Geometry check sheet. Reference: the model listing, model coordinates, mm. Face numbers are marked on the shaded views. A direction names the side the tool comes from. Round coordinates to 2 decimals unless told otherwise and drop trailing zeros. Loops run counter-clockwise (first coordinate to the right, second up) from the corner with the lowest first, then second, coordinate; pieces in that order, holes last. Notation, with made-up numbers: (6.25, -31) -> (24.25, -31) arc R27 cw to (24.25, -3) -> close; hole circle Ø2 at (50.5, 24.5). An arc over 180 degrees is marked (long way). Use a Markdown table: item, result. Add a question column.
Q1. Sectioned sample at A-A, the plane y = 150.75. Enter the section's corners in (x, z), then the cut area to 3 significant figures.
Q2. Sectioned sample at C-C, the plane x = 502.5. Enter the section's corners in (y, z).
Q3. Material ranges on L1, parallel to Z at x = 481.5, y = 149.5; L2, parallel to Y at x = 506, z = -18; L3, parallel to Z at x = 495, y = 142.5, recorded low to high.
Q4. Sectioned sample at B-B, the plane z = 21.5. Enter the section's corners in (x, y).
Q5. Gauge pin test, flat ends, axial feed: P1, Ø8.5, axis at x = 484.35, y = 151, coming from the -Z side; P2, Ø4, axis at x = 524, y = 136.5, coming from the +Z side; P3, Ø2, axis at y = 137, z = -47.5, coming from the +X side; P4, Ø4, axis at x = 522.92, z = -75.05, coming from the +Y side. Record the tip position at first contact, or that the pin passes through.
Q6. Set-up check for the marked faces 1 and 2: record each of +Z, -Z, +X, -X, +Y, -Y from which the full face is reachable in a straight line by a thin tool's end or side.
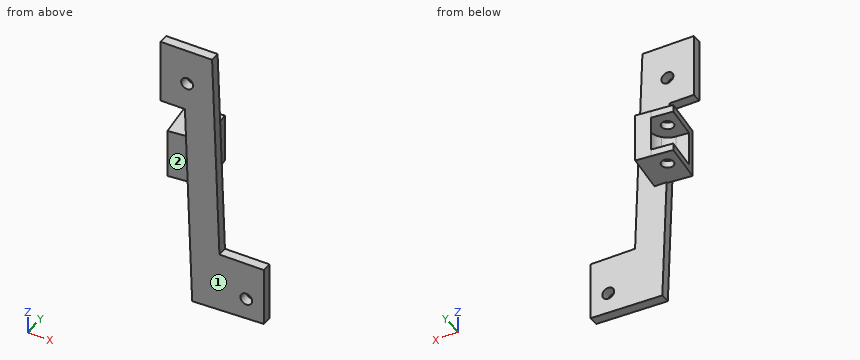
```python
from build123d import *

# Parameters (mm, degrees)
BOSS_EXTRUDE5_DEPTH = 22.352
BOSS_EXTRUDE7_START = -3.81
SKETCH2_R           = 3.175
BOSS_EXTRUDE7_DEPTH = 3.81
BOSS_EXTRUDE8_START = 3.81
SKETCH3_R           = 3.175
BOSS_EXTRUDE8_DEPTH = 3.81
BOSS_EXTRUDE9_DEPTH = 5.08
SKETCH6_R           = 3.175
CUT_EXTRUDE1_DEPTH  = 6.35


with BuildPart() as part:
    # Sketch1 → Boss-Extrude5 (new body)
    with BuildSketch(Plane.XY):
        with BuildLine():
            Line((485.284620904, 141.520479852), (478.661596161, 140.870936716))
            Line((478.661596161, 140.870936716), (479.033472001, 137.079128657))
            Line((479.033472001, 137.079128657), (498.224726786, 138.961281946))
            Line((498.224726786, 138.961281946), (496.114951182, 160.473473003))
            Line((496.114951182, 160.473473003), (488.231748542, 159.700339826))
            ThreePointArc((488.231748542, 159.700339826), (489.092376455, 159.263306748), (489.904354663, 158.741416237))
            ThreePointArc((489.904354663, 158.741416237), (493.83445145, 151.929689602), (491.302607825, 144.484217934))
            ThreePointArc((491.302607825, 144.484217934), (488.563156596, 142.455032775), (485.284620904, 141.520479852))
        make_face()
    extrude(amount=-BOSS_EXTRUDE5_DEPTH)

    # Sketch2 → Boss-Extrude7 (add)
    with BuildSketch(Plane(origin=(0, 0, -22.352), x_dir=(-1, 0, 0), z_dir=(0, 0, -1)).offset(BOSS_EXTRUDE7_START)):
        with BuildLine():
            Line((-476.923696397, 158.591319714), (-478.661596161, 140.870936716))
            Line((-478.661596161, 140.870936716), (-485.284620904, 141.520479852))
            ThreePointArc((-485.284620904, 141.520479852), (-493.757189232, 149.475804861), (-488.231748542, 159.700339826))
            Line((-488.231748542, 159.700339826), (-476.923696397, 158.591319714))
        make_face()
        with Locations(Location((-484.354931302, 151, 0), (0, 0, 90))):
            Circle(SKETCH2_R, mode=Mode.SUBTRACT)
    extrude(amount=BOSS_EXTRUDE7_DEPTH)

    # Sketch3 → Boss-Extrude8 (add)
    # profile 1 of 2: a face of its own
    with BuildSketch(Plane.XY.offset(BOSS_EXTRUDE8_START)):
        with BuildLine():
            Line((488.231748542, 159.700339826), (476.923696397, 158.591319714))
            Line((476.923696397, 158.591319714), (478.661596161, 140.870936716))
            Line((478.661596161, 140.870936716), (485.284620904, 141.520479852))
            ThreePointArc((485.284620904, 141.520479852), (493.757189232, 149.475804861), (488.231748542, 159.700339826))
        make_face()
        with Locations(Location((484.354931302, 151, 0), (0, 0, 90))):
            Circle(SKETCH3_R, mode=Mode.SUBTRACT)
    # profile 2 of 2: a face of its own
    with BuildSketch(Plane.XY.offset(BOSS_EXTRUDE8_START)):
        with BuildLine():
            Line((496.114951182, 160.473473003), (488.231748542, 159.700339826))
            ThreePointArc((488.231748542, 159.700339826), (493.757189232, 149.475804861), (485.284620904, 141.520479852))
            Line((485.284620904, 141.520479852), (478.661596161, 140.870936716))
            Line((478.661596161, 140.870936716), (479.033472001, 137.079128657))
            Line((479.033472001, 137.079128657), (498.224726786, 138.961281946))
            Line((498.224726786, 138.961281946), (496.114951182, 160.473473003))
        make_face()
    extrude(amount=-BOSS_EXTRUDE8_DEPTH)

    # Sketch4 → Boss-Extrude9 (add)
    with BuildSketch(Plane(origin=(0, 138.961281946, 0), x_dir=(1, 0, 0), z_dir=(0, 1, 0))):
        Polygon((494.072487043, 87.311338989), (532.291432121, 85.970092731), (532.291432121, 54.640280545), (508.611718184, 54.640280545), (504.692489504, -57.038529169), (477.269374414, -57.038529169), (477.269374414, -22.86), (490.206161169, -22.86), align=None)
    extrude(amount=-BOSS_EXTRUDE9_DEPTH)

    # Sketch6 → Cut-Extrude1 (cut)
    with BuildSketch(Plane(origin=(0, 138.961281946, 0), x_dir=(1, 0, 0), z_dir=(0, 1, 0))):
        with Locations(Location((491.366130704, -38.105065935, 0), (0, 0, 270))):
            Circle(SKETCH6_R)
        with Locations(Location((522.91714349, 75.049167666, 0), (0, 0, 270))):
            Circle(SKETCH6_R)
    extrude(amount=-CUT_EXTRUDE1_DEPTH, mode=Mode.SUBTRACT)


solid = part.part
```
Values:
| question | item | result |
|---|---|---|
| 1 | outline | (477.69, -22.35) -> (481.19, -22.35) -> (481.19, -18.54) -> (477.69, -18.54) -> close; (477.69, 0) -> (481.19, 0) -> (481.19, 3.81) -> (477.69, 3.81) -> close; (487.52, -22.35) -> (497.07, -22.35) -> (497.07, 3.81) -> (487.52, 3.81) -> (487.52, 0) -> (493.88, 0) -> (493.88, -18.54) -> (487.52, -18.54) -> close |
| 1 | area | 159 mm^2 |
| 2 | outline | (133.88, -87.02) -> (138.96, -87.02) -> (138.96, 57.04) -> (133.88, 57.04) -> close |
| 3 | L1 | -22.35 to -18.54, 0 to 3.81 |
| 3 | L2 | 133.88 to 138.96 |
| 3 | L3 | -22.35 to 3.81 |
| 4 | outline | (490.25, 133.88) -> (505.94, 133.88) -> (505.94, 138.96) -> (490.25, 138.96) -> close |
| 5 | P1 | z = -22.35 |
| 5 | P2 | z = -54.64 |
| 5 | P3 | x = 508.4 |
| 5 | P4 | through |
| 6 | face 1 | +Z, -Z, +X, -X, -Y |
| 6 | face 2 | -Z, -Y |
